```python
from build123d import *

# Parameters (mm, degrees)
PAD010_DEPTH  = 6
SKETCH038_R   = 1.1
HOLE011_DEPTH = 25
SKETCH039_R   = 1.1
HOLE012_DEPTH = 25
SKETCH052_R   = 0.8
HOLE019_DEPTH = 25


with BuildPart() as lift:
    # Sketch037 → Pad010 (new body)
    with BuildSketch(Plane.XY):
        with BuildLine():
            Line((-32.57, 26.255), (-32.57, 25.925))
            Line((-32.57, 25.925), (-34, 25.165))
            Line((-34, 25.165), (-34, 25.015))
            Line((-34, 25.015), (-32.57, 24.255))
            Line((-32.57, 24.255), (-32.57, 23.925))
            Line((-32.57, 23.925), (-34, 23.165))
            Line((-34, 23.165), (-34, 23.015))
            Line((-34, 23.015), (-32.57, 22.255))
            Line((-32.57, 22.255), (-32.57, 21.925))
            Line((-32.57, 21.925), (-34, 21.165))
            Line((-34, 21.165), (-34, 21.015))
            Line((-34, 21.015), (-32.57, 20.255))
            Line((-32.57, 20.255), (-32.57, 19.925))
            Line((-32.57, 19.925), (-34, 19.165))
            Line((-34, 19.165), (-34, 19.015))
            Line((-34, 19.015), (-32.57, 18.255))
            Line((-32.57, 18.255), (-32.57, 17.925))
            Line((-32.57, 17.925), (-34, 17.165))
            Line((-34, 17.165), (-34, 17.015))
            Line((-34, 17.015), (-32.57, 16.255))
            Line((-32.57, 16.255), (-32.57, 15.925))
            Line((-32.57, 15.925), (-34, 15.165))
            Line((-34, 15.165), (-34, 15.015))
            Line((-34, 15.015), (-32.57, 14.255))
            Line((-32.57, 14.255), (-32.57, 13.925))
            Line((-32.57, 13.925), (-34, 13.165))
            Line((-34, 13.165), (-34, 13.015))
            Line((-34, 13.015), (-32.57, 12.255))
            Line((-32.57, 12.255), (-32.57, 11.925))
            Line((-32.57, 11.925), (-34, 11.165))
            Line((-34, 11.165), (-34, 11.015))
            Line((-34, 11.015), (-32.57, 10.255))
            Line((-32.57, 10.255), (-32.57, 9.925))
            Line((-32.57, 9.925), (-34, 9.165))
            Line((-34, 9.165), (-34, 9.015))
            Line((-34, 9.015), (-32.57, 8.255))
            Line((-32.57, 8.255), (-32.57, 7.925))
            Line((-32.57, 7.925), (-34, 7.165))
            Line((-34, 7.165), (-34, 7.015))
            Line((-34, 7.015), (-32.57, 6.255))
            Line((-32.57, 6.255), (-32.57, 5.925))
            Line((-32.57, 5.925), (-34, 5.165))
            Line((-34, 5.165), (-34, 5.015))
            Line((-34, 5.015), (-32.57, 4.255))
            Line((-32.57, 4.255), (-32.57, 3.925))
            Line((-32.57, 3.925), (-34, 3.165))
            Line((-34, 3.165), (-34, 3.015))
            Line((-34, 3.015), (-32.57, 2.255))
            Line((-32.57, 2.255), (-32.57, 1.925))
            Line((-32.57, 1.925), (-34, 1.165))
            Line((-34, 1.165), (-34, 1.015))
            Line((-34, 1.015), (-32.57, 0.255))
            Line((-32.57, 0.255), (-32.57, -0.075))
            Line((-32.57, -0.075), (-34, -0.835))
            Line((-34, -0.835), (-34, -0.985))
            Line((-34, -0.985), (-32.57, -1.745))
            Line((-32.57, -1.745), (-32.57, -2.075))
            Line((-32.57, -2.075), (-34, -2.835))
            Line((-34, -2.835), (-34, -2.985))
            Line((-34, -2.985), (-32.57, -3.745))
            Line((-32.57, -3.745), (-32.57, -4.075))
            Line((-32.57, -4.075), (-34, -4.835))
            Line((-34, -4.835), (-34, -4.985))
            Line((-34, -4.985), (-32.57, -5.745))
            Line((-32.57, -5.745), (-32.57, -6.075))
            Line((-32.57, -6.075), (-34, -6.835))
            Line((-34, -6.835), (-34, -6.985))
            Line((-34, -6.985), (-32.57, -7.745))
            Line((-32.57, -7.745), (-32.57, -8.075))
            Line((-32.57, -8.075), (-34, -8.835))
            Line((-34, -8.835), (-34, -8.985))
            Line((-34, -8.985), (-32.57, -9.745))
            Line((-32.57, -9.745), (-32.57, -10.075))
            Line((-32.57, -10.075), (-34, -10.835))
            Line((-34, -10.835), (-34, -10.985))
            Line((-34, -10.985), (-32.57, -11.745))
            Line((-32.57, -11.745), (-32.57, -12.075))
            Line((-32.57, -12.075), (-34, -12.835))
            Line((-34, -12.835), (-34, -12.985))
            Line((-34, -12.985), (-32.57, -13.745))
            Line((-32.57, -13.745), (-32.57, -14.075))
            Line((-32.57, -14.075), (-34, -14.835))
            Line((-34, -14.835), (-34, -14.985))
            Line((-34, -14.985), (-32.57, -15.745))
            Line((-32.57, -15.745), (-32.57, -16.075))
            Line((-32.57, -16.075), (-34, -16.835))
            Line((-34, -16.835), (-34, -16.985))
            Line((-34, -16.985), (-32.57, -17.745))
            Line((-32.57, -17.745), (-32.57, -18.075))
            Line((-32.57, -18.075), (-34, -18.835))
            Line((-34, -18.835), (-34, -18.985))
            Line((-34, -18.985), (-32.57, -19.745))
            Line((-32.57, -19.745), (-32.57, -20.075))
            Line((-32.57, -20.075), (-34, -20.835))
            Line((-34, -20.835), (-34, -20.985))
            Line((-34, -20.985), (-32.57, -21.745))
            Line((-32.57, -21.745), (-32.57, -22.075))
            Line((-32.57, -22.075), (-34, -22.835))
            Line((-34, -22.835), (-34, -22.985))
            Line((-34, -22.985), (-32.57, -23.745))
            Line((-32.57, -23.745), (-32.57, -24.075))
            Line((-32.57, -24.075), (-34, -24.835))
            Line((-34, -24.835), (-34, -24.985))
            Line((-34, -24.985), (-32.57, -25.745))
            Line((-32.57, -25.745), (-32.57, -26.075))
            Line((-32.57, -26.075), (-34, -26.835))
            Line((-34, -26.835), (-34, -26.985))
            Line((-34, -26.985), (-32.57, -27.745))
            Line((-32.57, -27.745), (-32.57, -28.075))
            Line((-32.57, -28.075), (-34, -28.835))
            Line((-34, -28.835), (-34, -28.985))
            Line((-34, -28.985), (-32.57, -29.745))
            Line((-32.57, -29.745), (-32.57, -30.075))
            Line((-32.57, -30.075), (-34, -30.835))
            Line((-34, -30.835), (-34, -30.985))
            Line((-34, -30.985), (-32.57, -31.745))
            Line((-32.57, -31.745), (-32.57, -32.075))
            Line((-32.57, -32.075), (-34, -32.835))
            Line((-34, -32.835), (-34, -32.985))
            Line((-34, -32.985), (-32.57, -33.745))
            Line((-32.57, -33.745), (-32.57, -34.075))
            Line((-32.57, -34.075), (-34, -34.835))
            Line((-34, -34.835), (-34, -34.985))
            Line((-34, -34.985), (-32.57, -35.745))
            Line((-32.57, -35.745), (-32.57, -36.075))
            Line((-32.57, -36.075), (-34, -36.835))
            Line((-34, -36.835), (-34, -36.985))
            Line((-34, -36.985), (-32.57, -37.745))
            Line((-32.57, -37.745), (-32.57, -38.075))
            Line((-32.57, -38.075), (-34, -38.835))
            Line((-34, -38.835), (-34, -38.985))
            Line((-34, -38.985), (-32.57, -39.745))
            Line((-32.57, -39.745), (-32.57, -40.075))
            Line((-32.57, -40.075), (-34, -40.835))
            Line((-34, -40.835), (-34, -40.985))
            Line((-34, -40.985), (-32.57, -41.745))
            Line((-32.57, -41.745), (-32.57, -42.075))
            Line((-32.57, -42.075), (-34, -42.835))
            Line((-34, -42.835), (-34, -42.985))
            Line((-34, -42.985), (-32.57, -43.745))
            Line((-32.57, -43.745), (-32.57, -44.075))
            Line((-32.57, -44.075), (-34, -44.835))
            ThreePointArc((-34, -44.835), (-32.121614, -47.676332), (-29.038942, -49.125))
            Line((-29.038942, -49.125), (-29.038942, -111.835))
            Line((-56.038942, -111.835), (-29.038942, -111.835))
            Line((-56.038942, 27.015), (-56.038942, -111.835))
            Line((-34, 27.015), (-56.038942, 27.015))
            Line((-34, 27.015), (-32.57, 26.255))
        make_face()
    extrude(amount=PAD010_DEPTH)

    # Sketch038 (on Face150 of Pad010) → Hole011 (cut)
    with BuildSketch(Plane.XY.offset(6)):
        with Locations((-48, -69.585)):
            Circle(SKETCH038_R)
        with Locations((-36, -69.585)):
            Circle(SKETCH038_R)
        with Locations((-48, -82.585)):
            Circle(SKETCH038_R)
        with Locations((-36, -82.585)):
            Circle(SKETCH038_R)
    extrude(amount=-HOLE011_DEPTH, mode=Mode.SUBTRACT)

    # Sketch039 (on Face5 of Hole011) → Hole012 (cut)
    with BuildSketch(Plane.XY.offset(6)):
        with Locations((-53.038942, -108.835)):
            Circle(SKETCH039_R)
        with Locations((-46.038942, -108.835)):
            Circle(SKETCH039_R)
        with Locations((-39.038942, -108.835)):
            Circle(SKETCH039_R)
        with Locations((-32.038942, -108.835)):
            Circle(SKETCH039_R)
    extrude(amount=-HOLE012_DEPTH, mode=Mode.SUBTRACT)

    # Sketch052 (on Face5 of Hole012) → Hole019 (cut)
    with BuildSketch(Plane.XY.offset(6)):
        with Locations((-46, -9.33)):
            Circle(SKETCH052_R)
        with Locations((-38, -9.33)):
            Circle(SKETCH052_R)
        with Locations((-46, -17.33)):
            Circle(SKETCH052_R)
        with Locations((-38, -17.33)):
            Circle(SKETCH052_R)
    extrude(amount=-HOLE019_DEPTH, mode=Mode.SUBTRACT)


with BuildPart() as part_mirroring:
    # Part__Mirroring: instance of Lift
    add(lift.part.mirror(Plane(origin=(0, 0, 0), x_dir=(0, -1, 0), z_dir=(1, 0, 0))))


with BuildPart() as part_mirroring_1:
    # Part__Mirroring placement: moved
    add(part_mirroring.part.moved(Location((-56, 0, 16))))


solid = part_mirroring_1.part
```
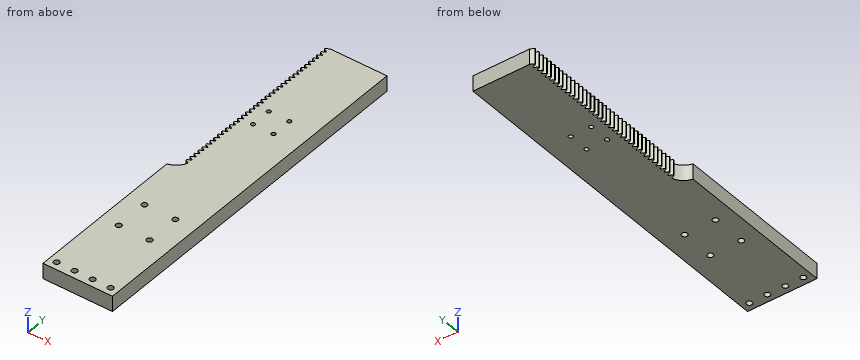
Check sheet for the modelled part. Datum: model origin and axes. Units: mm. Coordinates: 2 decimals unless noted, no trailing zeros. Use one line per item in the form item = value.
Item 1: Sectioned sample at A-A, the plane z = 20.15. State how many separate pieces and enclosed holes the cut face has, and give its area (3 significant figures).
Answer below:
separate_pieces = 1
enclosed_holes = 12
area = 3,400 mm^2
Item 2: Gauge pin test, flat end, axial feed: pin 1 Ø3 at (y, z) = (5, 20.5) entering from -X. Record the tip position at first contact, or that the pin passes through.
Answer below:
pin_1 = -23.43
Item 3: Material ranges on L1, parallel to Y at x = -10, z = 19.35 (3 decimals); L2, parallel to Y at x = -9.5, z = 16.7 (1 decimal); L3, parallel to Y at x = -7.5, z = 19.6 (3 decimals), recorded low to high. Write a range as from..to.
Answer below:
L1 = -111.835..-109.934, -107.736..-18.13, -16.53..-10.13, -8.53..27.015
L2 = -111.8..-109.8, -107.8..-18, -16.7..-10, -8.7..27
L3 = -111.835..-83.565, -81.605..-70.565, -68.605..27.015
